from build123d import *

# Parameters (mm, degrees)
SKETCH2_R           = 30.1625
BOSS_EXTRUDE1_DEPTH = 7.62
SCALE1_SCALE        = 0.41


with BuildPart() as part:
    # Sketch1 → Revolve1 (revolve)
    with BuildSketch(Plane.XY, mode=Mode.PRIVATE) as revolve1_sk:
        Polygon((-21.209, -30.1625), (21.209, -30.1625), (21.209, 0), (13.589, 0), (13.589, -26.2509), (-21.209, -26.2509), align=None)
    revolve(revolve1_sk.sketch.rotate(Axis((-21.209, 0, 0), (1, 0, 0)), 270), axis=Axis((-21.209, 0, 0), (1, 0, 0)))

    # Sketch2 → Boss-Extrude1 (add)
    with BuildSketch(Plane(origin=(21.209, 0, 0), x_dir=(0, 0, -1), z_dir=(1, 0, 0))):
        Polygon((-12.658107583, 30.559375), (-30.559375, 12.658107583), (-30.559375, -12.658107583), (-12.658107583, -30.559375), (12.658107583, -30.559375), (30.559375, -12.658107583), (30.559375, 12.658107583), (12.658107583, 30.559375), align=None)
        with Locations(Location((0, 0, 0), (0, 0, 180))):
            Circle(SKETCH2_R, mode=Mode.SUBTRACT)
    extrude(amount=-BOSS_EXTRUDE1_DEPTH)


with BuildPart() as part_1:
    # Scale1: scaled about (6.673848972, 0, 0)
    add(part.part.scale(SCALE1_SCALE).moved(Location((3.937570893, 0, 0))))


solid = part_1.part
CAD build for the part. Positions are in the model's coordinates, mm. A direction names the side the tool comes from. Coordinates: 2 decimals unless noted, no trailing zeros. Order: outer loops, then holes, each group sorted by start corner. A loop starts at its lowest first (then second) coordinate and runs counter-clockwise, first axis right, second up. Notation, with made-up numbers: (-22.5, 13) -> (29.5, 13) arc R19 ccw to (29.5, 44) -> close; hole circle Ø6 at (-4, -13). An arc over 180 degrees is marked (long way). Answer in a Markdown table with one row per item.
1) Band-saw the part on A-A (z = 0). List the corners of the cut face in (x, y), and give its area (3 significant figures).
Check values:
| item | result |
|---|---|
| outline | (-4.76, -12.37) -> (9.51, -12.37) -> (9.51, -12.53) -> (12.63, -12.53) -> (12.63, 12.53) -> (9.51, 12.53) -> (9.51, 12.37) -> (-4.76, 12.37) -> (-4.76, 10.76) -> (9.51, 10.76) -> (9.51, -10.76) -> (-4.76, -10.76) -> close |
| area | 124 mm2 |
2) Band-saw the part on C-C (y = 5.75). List the corners of the cut face in (x, z).
Check values:
| item | result |
|---|---|
| outline | (-4.76, -10.95) -> (9.51, -10.95) -> (9.51, -11.97) -> (12.63, -11.97) -> (12.63, 11.97) -> (9.51, 11.97) -> (9.51, 10.95) -> (-4.76, 10.95) -> (-4.76, 9.1) -> (9.51, 9.1) -> (9.51, -9.1) -> (-4.76, -9.1) -> close |
3) Mould opens along Z. For faces 1 (the face through (2.475, -8.358, -9.115)), 2 (the face through (9.509, 0, 0)), 3 (the face through (11, 12.529, 0)) say: pulls with the +Z half, pulls with the -Z half, needs draft (parallel to the pull), parting line crosses it, or undercut.
Check values:
| item | result |
|---|---|
| face 1 | parting line crosses it |
| face 2 | undercut |
| face 3 | needs draft |
4) Band-saw the part on B-B (x = 1.25). List the corners of the cut face in (y, z), and give its area (3 significant figures).
Check values:
| item | result |
|---|---|
| outline | circle Ø24.73 at (0, 0); hole circle Ø21.53 at (0, 0) |
| area | 117 mm2 |
5) Which spindle directions (+Z, -Z, +X, -X, +Y, -Y) get a long thin tool onto all of the face, cutting with end or side? Do faces 4 (the face through (11, -12.529, 0)), 5 (the face through (9.509, -11, -6)). Say none if no direction does.
Check values:
| item | result |
|---|---|
| face 4 | +Z, -Z, +X, -X, -Y |
| face 5 | -X |
6) Flat gauge pins, fed straight in: P1, Ø1, axis at x = 0.5, y = 4.5, coming from the -Z side; P2, Ø1, axis at x = -2.5, z = -10, coming from the +Y side; P3, Ø1.5, axis at x = 0.5, z = 4, coming from the +Y side. Where does each tip first touch, or does it go through?
Check values:
| item | result |
|---|---|
| P1 | z = -11.7 |
| P2 | y = 7.92 |
| P3 | y = 11.93 |
7) Drill centre lines: line 1 (Y direction, x = -0.5, z = 0); line 2 (X direction, y = -1.5, z = 5.5); line 3 (Z direction, x = 4, y = 9.75). Where is each one in solid material? Low to high.
Check values:
| item | result |
|---|---|
| line 1 | -12.37 to -10.76, 10.76 to 12.37 |
| line 2 | 9.51 to 12.63 |
| line 3 | -7.61 to -4.56, 4.56 to 7.61 |
